Verification items for the finished model (mm, model axes). A direction names the side the tool comes from. Coordinates: 2 decimals unless noted, no trailing zeros. Order: outer loops, then holes, each group sorted by start corner. A loop starts at its lowest first (then second) coordinate and runs counter-clockwise, first axis right, second up. Notation, with made-up numbers: M 33,35 L 89,35 A29 cw 89,58 Z; hole C 44.25,76.25 d1. An arc over 180 degrees is marked long. Answer as a JSON object with one key per item and string values. Group by question number.
(1) Access from +Z, -Z, +X, -X, +Y, -Y to the whole of each face (thin tool, end or side, straight path). Record for faces 5 (the face through (14, 8.805, 8)), 6 (the face through (-2.69, 11.74, 10.11)), 7 (the face through (14, -8.943, 8)).
(2) Cross-section at A-A (y = -6). Enter the section's corners in (x, z).
(3) Cross-section at C-C (z = 10.25). Enter the section's corners in (x, y).
(4) Gauge pin test, flat ends, axial feed: pin 1 Ø5 at (x, y) = (14, -7.5) entering from -Z; pin 2 Ø10 at (x, y) = (-3, 7.5) entering from +Z; pin 3 Ø5.5 at (x, z) = (-15, -54) entering from -Y; pin 4 Ø2 at (x, z) = (-16, -92) entering from +Y. Record the tip position at first contact, or that the pin passes through.
(5) Material ranges on line 1 (Y direction, x = -10.5, z = -92); line 2 (Z direction, x = 8.5, y = 5); line 3 (X direction, y = -0.25, z = -123), recorded low to high.
(6) Cross-section at D-D (z = -23). Enter the section's corners in (x, y), plus the area to 3 significant figures.
(7) Cross-section at B-B (x = -4). Enter the section's corners in (y, z).
(8) Mould release check, pull along X, two halves, no side actions. Record for faces 1 (the face through (11.963, 6.587, 10.851)), 2 (the face through (-2.613, -11.765, 10.106)), 3 (the face through (19.514, 7, 10)), 4 (the face through (11.963, -6.662, 10.851)): released by +X, released by -X, zero draft, split by the parting line, or undercut.
Autodesk Fusion 360 part; units mm, degrees
sketch "Sketch1" plane through (0, 0, 0) normal (0, 0, 1) x (1, 0, 0)
  line L0 (-6.8161, 4.6338) -> (-18.242, 4.6338)
  line L1 (8.001, -8.943) -> (19.5137, -8.943)
  line L2 (19.5137, -8.943) -> (19.5137, -4.443)
  line L3 (-18.242, -4.3662) -> (-6.9956, -4.3662)
  circle A0 centre (0.0069, -0.0041) radius 8.25
  arc A1 (-6.9956, -4.3662) -> (6.9609, -4.443) centre (0.0069, -0.0041) ccw
  line L4 (8.1435, 8.8053) -> (19.5137, 8.8053)
  line L5 (-11.0521, 4.6338) -> (-6.8161, 4.6338)
  line L6 (19.5137, 8.8053) -> (8.1435, 8.8053)
  line L7 (19.5137, -8.943) -> (19.5137, -4.443)
  arc A2 (-6.8161, 4.6338) -> (-6.9956, -4.3662) centre (0.0069, -0.0041) ccw
  line L8 (19.5137, 4.3053) -> (19.5137, 8.8053)
  line L9 (19.5137, 4.3053) -> (7.0419, 4.3053)
  circle A3 centre (0.0069, -0.0041) radius 12.0488
  line L10 (-18.242, 4.6338) -> (-18.242, -4.3662)
  line L11 (8.001, -8.943) -> (19.5137, -8.943)
  line L12 (19.5137, 4.3053) -> (19.5137, 8.8053)
  arc A4 (7.0419, 4.3053) -> (-6.8161, 4.6338) centre (0.0069, -0.0041) ccw
  line L13 (7.0419, 4.3053) -> (19.5137, 4.3053)
  line L14 (19.5137, -4.443) -> (6.9609, -4.443)
  line L15 (-11.0521, 4.6338) -> (-18.242, 4.6338)
  line L16 (-6.9956, -4.3662) -> (-11.1637, -4.3662)
  line L17 (-18.242, -4.3662) -> (-11.1637, -4.3662)
  line L18 (-18.242, 4.6338) -> (-18.242, -4.3662)
  line L19 (0.0069, -0.0041) -> (-18.242, -0.0041) construction
  line L20 (-8.2415, 0.1604) -> (-8.2415, -4.3662)
  line L21 (-8.2415, 0.1604) -> (-8.2415, 4.6355)
  line L22 (-8.2415, -4.3662) -> (-8.2415, 4.6355)
  dimension "d6" = 90
extrude "Extrude1" add sketch "Sketch1" along normal blind 20.5 contours L0 A0 L5 A2 L21 L22 | L0 A0 L5 L9 A3 A4 L13 L15 | L3 A0 A2 L16 L20 L22 | L0 L3 L5 A3 L15 L16 L17 L20 L21 L22 | L4 L6 L8 L9 A3 L12 L13 | L3 A0 A1 A3 L14 L16 L17 | L0 L3 A3 L10 L15 L17 L18 | L1 L2 L7 A3 L11 L14
sketch "Sketch2" plane through (0, 8.8053, 0) normal (0, 1, 0) x (-1, 0, 0)
  line L0 (-19.5137, 0) -> (-8.2268, 0)
  line L1 (-8.2268, 20.5) -> (-19.5137, 20.5)
  line L2 (-19.5137, 20.5) -> (-19.5137, 0)
  line L3 (-8.2268, 0) -> (-19.5137, 20.5) construction
  line L4 (-8.2268, 20.5) -> (-19.5137, 0) construction
  circle A0 centre (-13.8702, 10.25) radius 2
  line L5 (-8.2268, 0) -> (-8.2268, 20.5)
  dimension "d3" = 4
extrude "Extrude2" cut sketch "Sketch2" against normal blind 39 contours A0
extrude "Extrude3" add sketch "Sketch1" against normal blind 141.5 contours L0 L3 L5 A3 L15 L16 L17 L20 L21 L22 | L0 L3 A3 L10 L15 L17 L18
extrude "Extrude4" cut sketch "Sketch1" against normal blind 144 contours L0 A0 L5 A2 L21 L22 | L3 A0 A2 L16 L20 L22
extrude "Extrude5" cut 1 faces at (-9.3904, -2.3691, -141.5) along direction (0, 0, 1) blind 141
extrude "Extrude6" add 1 faces at (-9.3904, -2.3691, -0.5) along direction (0, 0, -1) blind 141
Taken from the geometry:
{
 "1": {"face 5": "+Z, -Z, +X, +Y", "face 6": "+Z, -Z, +Y", "face 7": "+Z, -Z, +X, -Y"},
 "2": {"outline": "M -10.44,0 L -5.66,0 L -5.66,20.5 L -10.44,20.5 Z; M 5.67,0 L 19.51,0 L 19.51,20.5 L 5.67,20.5 Z; hole C 13.87,10.25 d4"},
 "3": {"outline": "M -18.24,-4.37 L -11.22,-4.37 A12.05 ccw 8.09,-8.94 L 11.87,-8.94 L 11.87,-4.44 L 6.96,-4.44 A8.25 cw long 7.04,4.31 L 11.87,4.31 L 11.87,8.81 L 8.23,8.81 A12.05 ccw -11.11,4.63 L -18.24,4.63 Z; M 15.87,-8.94 L 19.51,-8.94 L 19.51,-4.44 L 15.87,-4.44 Z; M 15.87,4.31 L 19.51,4.31 L 19.51,8.81 L 15.87,8.81 Z"},
 "4": {"pin 1": "stops at z = 0", "pin 2": "stops at z = 20.5", "pin 3": "stops at y = -4.37", "pin 4": "stops at y = 4.63"},
 "5": {"line 1": "y = -4.37 to 4.63", "line 2": "z = 0 to 20.5", "line 3": "x = -18.24 to -8.24"},
 "6": {"outline": "M -18.24,-4.37 L -8.24,-4.37 L -8.24,4.64 L -18.24,4.63 Z", "area": "90.0 mm²"},
 "7": {"outline": "M -11.37,0 L -7.22,0 L -7.22,20.5 L -11.37,20.5 Z; M 7.21,0 L 11.36,0 L 11.36,20.5 L 7.21,20.5 Z"},
 "8": {"face 1": "undercut", "face 2": "split by the parting line", "face 3": "released by +X", "face 4": "undercut"}
}
